```python
from build123d import *

# Parameters (mm, degrees)
BOSS_EXTRUDE1_DEPTH                     = 22
BOSS_EXTRUDE1_DEPTH_BACK                = 22
BOSS_EXTRUDE3_DEPTH                     = 10
CUT_EXTRUDE2_DEPTH                      = 10
RIB1_REACH                              = 103.581
SKETCH4_WALL_W                          = 263.805794056
SKETCH4_WALL_H                          = 6
CBORE_FOR_M5_HEX_HEAD_BOLT1_D           = 6
CBORE_FOR_M5_HEX_HEAD_BOLT1_DEPTH       = 10
CBORE_FOR_M5_HEX_HEAD_BOLT1_CBORE_D     = 12
CBORE_FOR_M5_HEX_HEAD_BOLT1_CBORE_DEPTH = 3
CBORE_FOR_M5_HEX_HEAD_BOLT1_TIP         = 1.732050808
FILLET1_R                               = 10


with BuildPart() as part:
    # Sketch1 → Boss-Extrude1 (new, two sides: drawn at the far end of the back side and taken through both)
    with BuildSketch(Plane.XY.offset(-BOSS_EXTRUDE1_DEPTH_BACK)):
        Polygon((0, 0), (-63.773502692, 0), (-87.660254038, 41.373066959), (-79, 46.373066959), (-58, 10), (0, 10), align=None)
    extrude(amount=BOSS_EXTRUDE1_DEPTH + BOSS_EXTRUDE1_DEPTH_BACK)

    # Sketch3 → Boss-Extrude3 (add)
    with BuildSketch(Plane(origin=(0, 10, 0), x_dir=(1, 0, 0), z_dir=(0, 1, 0))):
        with BuildLine():
            Line((0, -6), (0, -22))
            ThreePointArc((0, -22), (22, 0), (0, 22))
            Line((0, 22), (0, 6))
            ThreePointArc((0, 6), (6, 0), (0, -6))
        make_face()
    extrude(amount=-BOSS_EXTRUDE3_DEPTH)

    # Sketch3_3 → Cut-Extrude2 (cut)
    with BuildSketch(Plane(origin=(0, 10, 0), x_dir=(1, 0, 0), z_dir=(0, 1, 0))):
        with BuildLine():
            Line((-25, -6), (0, -6))
            Line((0, -6), (0, 6))
            Line((0, 6), (-25, 6))
            ThreePointArc((-25, 6), (-31, 0), (-25, -6))
        make_face()
        with BuildLine():
            Line((0, 6), (0, -6))
            ThreePointArc((0, -6), (6, 0), (0, 6))
        make_face()
    extrude(amount=-CUT_EXTRUDE2_DEPTH, mode=Mode.SUBTRACT)

    # Sketch4 wall → Rib1 (add, up to next)
    with BuildSketch(Plane(origin=(-56, 28.186533479, 0), x_dir=(0.784407511397, -0.620245802939, 0), z_dir=(0.620245802939, 0.784407511397, 0)), mode=Mode.PRIVATE) as rib1_sk1:
        Rectangle(SKETCH4_WALL_W, SKETCH4_WALL_H)
    rib1_tool1 = extrude(rib1_sk1.sketch, amount=-RIB1_REACH, mode=Mode.PRIVATE) - part.part
    add(rib1_tool1.solids().sort_by_distance((-56, 28.186533479, 0))[0])

    # CBORE for M5 Hex Head Bolt1
    with Locations(Plane(origin=(-39.169872981, -22.61473671, 0), x_dir=(0, 0, -1), z_dir=(0.8660254037844395, 0.49999999999999856, 0))):
        with Locations((-12.5, 70.186913626), (12.5, 70.186913626)):
            CounterBoreHole(CBORE_FOR_M5_HEX_HEAD_BOLT1_D / 2, CBORE_FOR_M5_HEX_HEAD_BOLT1_CBORE_D / 2, CBORE_FOR_M5_HEX_HEAD_BOLT1_CBORE_DEPTH, depth=CBORE_FOR_M5_HEX_HEAD_BOLT1_DEPTH)
            with Locations((0, 0, -(CBORE_FOR_M5_HEX_HEAD_BOLT1_DEPTH + CBORE_FOR_M5_HEX_HEAD_BOLT1_TIP / 2))):  # 120° drill point
                Cone(0, CBORE_FOR_M5_HEX_HEAD_BOLT1_D / 2, CBORE_FOR_M5_HEX_HEAD_BOLT1_TIP, mode=Mode.SUBTRACT)

    # Fillet1
    fillet1_edges = [part.edges().sort_by_distance(p)[0] for p in [
        (-83.330127019, 43.873066959, -22),
        (-83.330127019, 43.873066959, 22),
    ]]
    fillet(fillet1_edges, radius=FILLET1_R)


solid = part.part
```
Read the model definition and answer for the solid it produces. Units are mm, in the model's axes. A direction names the side the tool comes from. Coordinates: 2 decimals unless noted, no trailing zeros. Write each loop counter-clockwise with the first axis right and the second up, starting at its lowest first coordinate (ties: lowest second). Pieces come first, ordered by that corner, then holes. Notation, with made-up numbers: (-32.5, 12.25) - (20.5, 12.25) arc R16 cw to (20.5, 27.25) - close; hole circle Ø1 at (24.25, -30.5). An arc over 180 degrees is marked (long way). Answer as a JSON object with one key per item and string values. Group by question number.
1. A cutting plane is placed at B-B (z = 0). Determine the outline of the cut face in (x, y), plus the area to 3 significant figures.
2. Each of these flat-tipped pins is pushed along its axis until it touches: P1, Ø6, axis at x = -36, z = -14.5, coming from the +Y side; P2, Ø5, axis at y = 22.5, z = 6.5, coming from the -X side; P3, Ø1.5, axis at x = -63.5, z = -3, coming from the +Y side. Where does it stop, or does it pass through?
3. A cutting plane is placed at A-A (x = -15.5). Determine the outline of the cut face in (y, z), plus the area to 3 significant figures.
4. The mould has two halves that part along Z. Classify faces 4 (the cylindrical face through (22, 5, 0)), 5 (the cylindrical face through (-79.02, 33.31, -14.88)), 6 (the flat face through (-83.39, 43.84, -0.17)), 7 (the cylindrical face through (-81.844, 41.438, -18.993)): +Z half, -Z half, draft (parallel to the pull), parting line (faces both ways), or undercut.
5. A cutting plane is placed at C-C (y = 6.5). Determine the outline of the cut face in (x, z), plus the area to 3 significant figures.
6. Consider L1, parallel to Y at x = -78.5, z = -13.5; L2, parallel to X at y = 3.5, z = 5; L3, parallel to Y at x = -2.5, z = -12. Determine where each line is inside the solid, lowest interval first. Write a range as [from, to].
7. A cutting plane is placed at D-D (y = 22). Determine the outline of the cut face in (x, z).
8. Which of the six approach directions +Z, -Z, +X, -X, +Y, -Y give full straight-line access (tool end or side, diameter ignored) to faces 1 (the cylindrical face through (-31, 5, 0)), 2 (the flat face through (-68.647, 28.441, -12.633)), 3 (the flat face through (-19, 10, 9))?
Worked out:
{
 "1": {"outline": "(-87.66, 41.37) - (-63.77, 0) - (-31, 0) - (-31, 10) - (-33, 10) - (-79, 46.37) - close; (6, 0) - (22, 0) - (22, 10) - (6, 10) - close", "area": "1,360 mm²"},
 "2": {"P1": "stops at y = 10", "P2": "stops at x = -78.21", "P3": "stops at y = 34.71"},
 "3": {"outline": "(0, -22) - (10, -22) - (10, -6) - (0, -6) - close; (0, 6) - (10, 6) - (10, 22) - (0, 22) - close", "area": "320 mm²"},
 "4": {"face 4": "parting line", "face 5": "undercut", "face 6": "draft", "face 7": "-Z half"},
 "5": {"outline": "(-67.53, -22) - (0, -22) arc R22 ccw to (0, 22) - (-67.53, 22) - close; hole (-25, -6) - (0, -6) arc R6 ccw to (0, 6) - (-25, 6) arc R6 ccw to start", "area": "3,320 mm²"},
 "6": {"L1": "y = [25.51, 32.46], [38.99, 39.51], [42.55, 45.51]", "L2": "x = [-65.79, -28.32], [3.32, 21.42]", "L3": "y = [0, 10]"},
 "7": {"outline": "(-76.48, -22) - (-64.93, -22) - (-64.93, -3) - (-48.18, -3) - (-48.18, 3) - (-64.93, 3) - (-64.93, 22) - (-76.48, 22) - close"},
 "8": {"face 1": "+Y, -Y", "face 2": "-Z, +X, +Y", "face 3": "+X, +Y"}
}
